Input: part model. Units: mm. Frame: model coordinates. A direction names the side the tool comes from. Coordinates: 2 decimals unless noted, no trailing zeros. Order: outer loops, then holes, each group sorted by start corner. A loop starts at its lowest first (then second) coordinate and runs counter-clockwise, first axis right, second up. Notation, with made-up numbers: M -29,46 L 20,46 A13 ccw 20,70 Z; hole C 12,44 d7. An arc over 180 degrees is marked long. One line per item, written item: value.
```python
from build123d import *

# Parameters (mm, degrees)
SKETCH2_R           = 15
BOSS_EXTRUDE2_DEPTH = 20
SKETCH3_R           = 30
SKETCH3_R_2         = 15
BOSS_EXTRUDE3_DEPTH = 10
SKETCH4_R           = 15
BOSS_EXTRUDE4_DEPTH = 70
FILLET1_R           = 5
FILLET2_R           = 5


with BuildPart() as part:
    # Sketch2 → Boss-Extrude2 (new body)
    with BuildSketch(Plane.XY):
        with BuildLine():
            Line((-100, -30), (100, -30))
            ThreePointArc((100, -30), (127.716385975, -11.480502971), (121.213203436, 21.213203436))
            Line((121.213203436, 21.213203436), (21.213203436, 121.213203436))
            ThreePointArc((21.213203436, 121.213203436), (0, 130), (-21.213203436, 121.213203436))
            Line((-21.213203436, 121.213203436), (-121.213203436, 21.213203436))
            ThreePointArc((-121.213203436, 21.213203436), (-127.716385975, -11.480502971), (-100, -30))
        make_face()
        with Locations((100, 0)):
            Circle(SKETCH2_R, mode=Mode.SUBTRACT)
        with Locations((-100, 0)):
            Circle(SKETCH2_R, mode=Mode.SUBTRACT)
        with Locations((0, 100)):
            Circle(SKETCH2_R, mode=Mode.SUBTRACT)
    extrude(amount=BOSS_EXTRUDE2_DEPTH)

    # Sketch3 → Boss-Extrude3 (add)
    # profile 1 of 3: a face of its own
    with BuildSketch(Plane.XY.offset(20)):
        with Locations(Location((-100, 0, 0), (0, 0, 135))):
            Circle(SKETCH3_R)
        with Locations((-100, 0)):
            Circle(SKETCH3_R_2, mode=Mode.SUBTRACT)
    # profile 2 of 3: a face of its own
    with BuildSketch(Plane.XY.offset(20)):
        with Locations(Location((100, 0, 0), (0, 0, 270))):
            Circle(SKETCH3_R)
        with Locations((100, 0)):
            Circle(SKETCH3_R_2, mode=Mode.SUBTRACT)
    # profile 3 of 3: a face of its own
    with BuildSketch(Plane.XY.offset(20)):
        with Locations(Location((0, 100, 0), (0, 0, 135))):
            Circle(SKETCH3_R)
        with Locations((0, 100)):
            Circle(SKETCH3_R_2, mode=Mode.SUBTRACT)
    extrude(amount=BOSS_EXTRUDE3_DEPTH)

    # Sketch4 → Boss-Extrude4 (add)
    with BuildSketch(Plane.XZ.offset(30)):
        with BuildLine():
            Line((20, 49.8), (20, 20))
            Line((20, 20), (-20, 20))
            Line((-20, 20), (-20, 49.8))
            ThreePointArc((-20, 49.8), (0, 69.8), (20, 49.8))
        make_face()
        with Locations(Location((0, 49.8, 0), (0, 0, 270))):
            Circle(SKETCH4_R, mode=Mode.SUBTRACT)
    extrude(amount=-BOSS_EXTRUDE4_DEPTH)

    # Fillet1
    fillet1_edges = [part.edges().sort_by_distance(p)[0] for p in [
        (20, 5, 20),
    ]]
    fillet(fillet1_edges, radius=FILLET1_R)

    # Fillet2
    fillet2_edges = [part.edges().sort_by_distance(p)[0] for p in [
        (-20, 5, 20),
    ]]
    fillet(fillet2_edges, radius=FILLET2_R)


solid = part.part
```
(1) Access query for faces 1 (the flat face through (-95, -15, 30)), 2 (the flat face through (0, 40, 34)), 3 (the flat face through (-5, 85, 30)), 4 (the flat face through (114, -6, 30)), 5 (the cylindrical face through (22, 5, 21)). Directions: +Z, -Z, +X, -X, +Y, -Y. A direction counts if a zero-diameter tool reaches every point of the face in a straight line with its end or side. Return the directions, or none.
Data:
face 1: +Z, -X, +Y, -Y
face 2: +Z, +X, -X
face 3: +Z, +X, -X, +Y
face 4: +Z, +X, +Y, -Y
face 5: +Z, -Y
(2) First-contact query: pin 1 (25 mm diameter, centred on x = 10.5, z = 36, fed in from +Y); pin 2 (12.5 mm diameter, centred on y = 3.5, z = 32, fed in from +X); pin 3 (6 mm diameter, centred on y = -5.5, z = 31.5, fed in from +X); pin 4 (2 mm diameter, centred on y = 32, z = 59.5, fed in from +X). Flat tips, straight axial feed; report the tip coordinate or a pass-through.
Data:
pin 1: stops at y = 130
pin 2: stops at x = 130
pin 3: stops at x = 129.86
pin 4: stops at x = 18.01
(3) Cut plane D-D on y = 81. Output: boundary loops of the cut face in (x, z).
Data:
outline: M -61.43,0 L 61.43,0 L 61.43,20 L 23.22,20 L 23.22,30 L -23.22,30 L -23.22,20 L -61.43,20 Z
(4) Cut plane A-A on x = 0. Output: boundary loops of the cut face in (y, z), plus the area to 3 significant figures.
Data:
outline: M -30,0 L 85,0 L 85,30 L 70,30 L 70,20 L 40,20 L 40,34.8 L -30,34.8 Z; M -30,64.8 L 40,64.8 L 40,69.8 L -30,69.8 Z; M 115,0 L 130,0 L 130,30 L 115,30 Z
area: 4,290 mm2
(5) Ray query, line 1 (Y direction, x = 0, z = 8); line 2 (Y direction, x = -100, z = 21); line 3 (Z direction, x = 76, y = 44.5). Return the intervals inside material, ascending. Write a range as from..to.
Data:
line 1: y = -30..85, 115..130
line 2: y = -30..-15, 15..30
line 3: z = 0..20
(6) Cut plane C-C on y = 100. Output: boundary loops of the cut face in (x, z).
Data:
outline: M -42.43,0 L -15,0 L -15,30 L -30,30 L -30,20 L -42.43,20 Z; M 15,0 L 42.43,0 L 42.43,20 L 30,20 L 30,30 L 15,30 Z
(7) Cut plane B-B on z = 38. Output: boundary loops of the cut face in (x, y), plus the area to 3 significant figures.
Data:
outline: M -20,-30 L -9.26,-30 L -9.26,40 L -20,40 Z; M 9.26,-30 L 20,-30 L 20,40 L 9.26,40 Z
area: 1,500 mm2
(8) Draft query along X for faces 6 (the flat face through (-2, 33, 0)), 7 (the cylindrical face through (-85.693, 4.506, 14.79)), 8 (the flat face through (71.913, 70.513, 9.86)). Return one class per face: released by +X, released by -X, zero draft, split by the parting line, or undercut.
Data:
face 6: zero draft
face 7: undercut
face 8: released by +X
